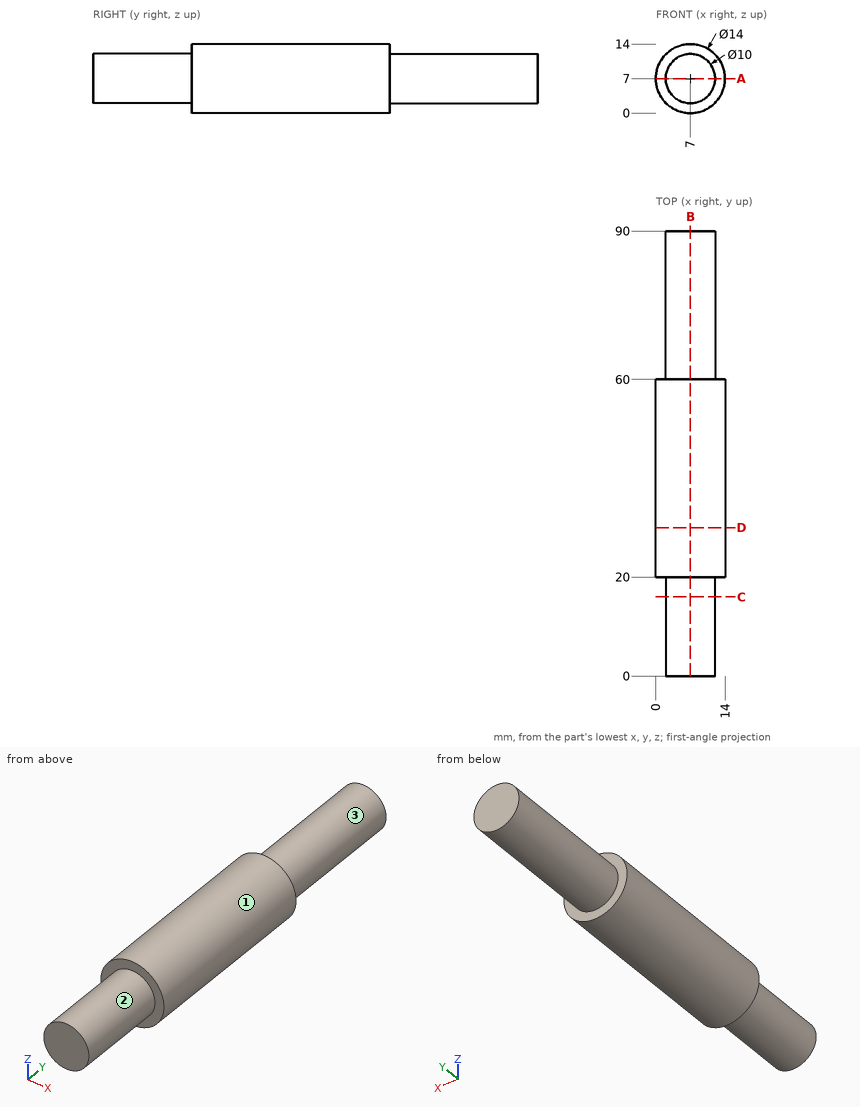
Answer from the drawing. Dimensions are ordinates in mm from the lowest x, y and z of the part. A direction names the side the tool comes from. Coordinates: 2 decimals unless noted, no trailing zeros. Write each loop counter-clockwise with the first axis right and the second up, starting at its lowest first coordinate (ties: lowest second). Pieces come first, ordered by that corner, then holes. Notation, with made-up numbers: M 57.25,69 L 98.25,69 A22 cw 98.25,108 Z; hole C 52,-11 d7. An arc over 180 degrees is marked long. Use one line per item in the form item = value. Start each with the question number.
1. The part is cut by section C-C (y = 16). Give the vertices of the cut face in (x, z), plus the area to 3 significant figures.
2. Straight lines are drawn through the part: probe 1 along Y at (x, z) = (9.25, 0.75); probe 2 along Z at (x, y) = (7, 66.5); probe 3 along X at (y, z) = (57.5, 10.75). For each, find the intervals that lie inside material, in ascending order. Write a range as from..to.
3. The part is cut by section A-A (z = 7). Give the vertices of the cut face in (x, y), plus the area to 3 significant figures.
4. Each of these flat-tipped pins is pushed along its axis until it touches: P1, Ø5, axis at x = 6.5, y = 80.5, coming from the -Z side; P2, Ø1, axis at x = 8, y = 47, coming from the +Z side; P3, Ø3, axis at x = 5, y = 60.5, coming from the -Z side. Where does it stop, or does it pass through?
5. The part is cut by section D-D (y = 30). Give the vertices of the cut face in (x, z), plus the area to 3 significant figures.
6. A tool of negligible diameter and unlimited length cuts with its end or side. For the marked faces 1, 2 and 3, from which of +Z, -Z, +X, -X, +Y, -Y can it reach the whole face along a straight path? Write none if from no direction.
7. The part is cut by section B-B (x = 7). Give the vertices of the cut face in (y, z), plus the area to 3 significant figures.
Evaluation:
q1.outline = C 7,7 d10
q1.area = 78.5 mm^2
q2.probe_1 = 20..60
q2.probe_2 = 2..12
q2.probe_3 = 1.09..12.91
q3.outline = M 0,20 L 2,20 L 2,0 L 12,0 L 12,20 L 14,20 L 14,60 L 12,60 L 12,90 L 2,90 L 2,60 L 0,60 Z
q3.area = 1,060 mm^2
q4.P1 = 2
q4.P2 = 13.98
q4.P3 = 0.02
q5.outline = C 7,7 d14
q5.area = 154 mm^2
q6.face_1 = +Y, -Y
q6.face_2 = -Y
q6.face_3 = +Y
q7.outline = M 0,2 L 20,2 L 20,0 L 60,0 L 60,2 L 90,2 L 90,12 L 60,12 L 60,14 L 20,14 L 20,12 L 0,12 Z
q7.area = 1,060 mm^2
